```python
from build123d import *

# Parameters (mm, degrees)
EXTRUDE_1_DEPTH     = 17
EXTRUDE_2_DEPTH     = 2
SKETCH_4_R          = 3.35
EXTRUDE_3_DEPTH     = 5
SKETCH_5_R          = 1.7
EXTRUDE_4_DEPTH     = 6.8
CUT_EXTRUDE_1_DEPTH = 5


with BuildPart() as part:
    # Эскиз1 → Бобышка-Вытянуть1 (new body)
    with BuildSketch(Plane(origin=(0, 0, 0), x_dir=(0, 0, -1), z_dir=(1, 0, 0))):
        with BuildLine():
            Line((-3.35, -2.3), (-3.35, 2.3))
            ThreePointArc((-3.35, 2.3), (0, 5.65), (3.35, 2.3))
            Line((3.35, 2.3), (3.35, -2.3))
            ThreePointArc((3.35, -2.3), (0, -5.65), (-3.35, -2.3))
        make_face()
    extrude(amount=-EXTRUDE_1_DEPTH)

    # Эскиз3 → Бобышка-Вытянуть2 (add)
    with BuildSketch(Plane.ZY):
        with BuildLine():
            Line((2.15, 2.35), (2.15, -2.35))
            ThreePointArc((2.15, -2.35), (0, -4.5), (-2.15, -2.35))
            Line((-2.15, -2.35), (-2.15, 2.35))
            ThreePointArc((-2.15, 2.35), (0, 4.5), (2.15, 2.35))
        make_face()
    extrude(amount=-EXTRUDE_2_DEPTH)

    # Эскиз4 → Бобышка-Вытянуть3 (add)
    with BuildSketch(Plane(origin=(-17, 0, 0), x_dir=(0, 0, -1), z_dir=(1, 0, 0))):
        Circle(SKETCH_4_R)
    extrude(amount=-EXTRUDE_3_DEPTH)

    # По траектории1: sweep along a path in Эскиз6
    with BuildLine(Plane.XY) as sweep_1_path:
        Line((-22, 0), (-24.776161806, 0))
        ThreePointArc((-24.776161806, 0), (-30.870449905, -0.986593903), (-36.342181829, -3.845591055))
    # Эскиз5 → По траектории1 (sweep)
    with BuildSketch(Plane.ZY.offset(22)):
        Circle(SKETCH_5_R)
    sweep(path=sweep_1_path.line)

    # Эскиз7 → Бобышка-Вытянуть4 (add)
    with BuildSketch(Plane(origin=(2, 0, 0), x_dir=(0, 0, -1), z_dir=(1, 0, 0))):
        with BuildLine():
            Line((-1.2, -2.925), (-1.2, 2.925))
            ThreePointArc((-1.2, 2.925), (0, 4.125), (1.2, 2.925))
            Line((1.2, 2.925), (1.2, -2.925))
            ThreePointArc((1.2, -2.925), (0, -4.125), (-1.2, -2.925))
        make_face()
    extrude(amount=EXTRUDE_4_DEPTH)

    # Эскиз8 → Вырез-Вытянуть1 (cut)
    with BuildSketch(Plane(origin=(8.8, 0, -8.8), x_dir=(0, 0, 1), z_dir=(-1, 0, 0))):
        with BuildLine():
            Line((8.25, -3.15), (8.25, 3.15))
            ThreePointArc((8.25, 3.15), (8.8, 3.7), (9.35, 3.15))
            Line((9.35, 3.15), (9.35, -3.15))
            ThreePointArc((9.35, -3.15), (8.8, -3.7), (8.25, -3.15))
        make_face()
    extrude(amount=CUT_EXTRUDE_1_DEPTH, mode=Mode.SUBTRACT)


solid = part.part
```
Input: part model. Units: mm. Frame: model coordinates. A direction names the side the tool comes from. Round coordinates to 2 decimals unless told otherwise and drop trailing zeros. Loops run counter-clockwise (first coordinate to the right, second up) from the corner with the lowest first, then second, coordinate; pieces in that order, holes last. Notation, with made-up numbers: (66.25, 3.5) -> (71.25, 3.5) arc R18 ccw to (71.25, 32.5) -> close; hole circle Ø5 at (40, -31.5). An arc over 180 degrees is marked (long way). Use one line per item in the form item = value. Start each with the question number.
Item 1: Mould query, pull axis Y, two halves, no side actions, for faces 1 (the face through (-23.41, -1.66, -0.37)), 2 (the face through (-8.38, -5.65, -0.07)), 3 (the face through (8.8, 0, -1)), 4 (the face through (6.3, 3.7, 0)). Classes: pulls with the +Y half, pulls with the -Y half, needs draft (parallel to the pull), parting line crosses it, or undercut.
Item 2: Section query B-B on x = -4. Return the cut outline in (y, z), then the cut area to 3 significant figures.
Item 3: Section query A-A on z = 0. Return the cut outline in (x, y) (3 decimals).
Item 4: Contact query for flat-ended pins moving along their axis: pin 1 Ø4.5 at (x, y) = (6, -0.5) entering from -Z; pin 2 Ø2.5 at (x, y) = (6, -1) entering from +Z; pin 3 Ø0.9 at (y, z) = (-1.5, 0) entering from +X. Output: stop coordinate, or through.
Item 5: Material intervals for L1, parallel to Z at x = 4, y = -2.5; L2, parallel to Z at x = 2.5, y = -2.75; L3, parallel to X at y = 0.75, z = 2.75, sorted ascending. Write a range as from..to.
Item 6: Set-up query: faces 5 (the face through (1, 4.5, 0)), 6 (the face through (-22, 1, 2)), 7 (the face through (5, 0, -1.2)), 8 (the face through (6.3, -3.7, 0)), 9 (the face through (1, 0, 2.15)). Return all of +Z, -Z, +X, -X, +Y, -Y with unobstructed straight access to the full face (end or side cutting, diameter ignored); none if empty.
Ans:
q1.face_1 = parting line crosses it
q1.face_2 = pulls with the -Y half
q1.face_3 = needs draft
q1.face_4 = undercut
q2.outline = (-2.3, -3.35) -> (2.3, -3.35) arc R3.35 ccw to (2.3, 3.35) -> (-2.3, 3.35) arc R3.35 ccw to start
q2.area = 66.1 mm^2
q3.outline = (-37.36, -2.484) -> (-35.324, -5.207) arc R17.616 cw to (-24.776, -1.7) -> (-22, -1.7) -> (-22, -3.35) -> (-17, -3.35) -> (-17, -5.65) -> (0, -5.65) -> (0, -4.5) -> (2, -4.5) -> (2, -4.125) -> (8.8, -4.125) -> (8.8, -3.7) -> (3.8, -3.7) -> (3.8, 3.7) -> (8.8, 3.7) -> (8.8, 4.125) -> (2, 4.125) -> (2, 4.5) -> (0, 4.5) -> (0, 5.65) -> (-17, 5.65) -> (-17, 3.35) -> (-22, 3.35) -> (-22, 1.7) -> (-24.776, 1.7) arc R21.016 ccw to start
q4.pin_1 = -1.2
q4.pin_2 = 1.2
q4.pin_3 = 3.8
q5.L1 = -1.2..-0.55, 0.55..1.2
q5.L2 = -1.2..1.2
q5.L3 = -22..0
q6.face_5 = +X, +Y
q6.face_6 = none
q6.face_7 = -Z, +X, +Y, -Y
q6.face_8 = +X
q6.face_9 = +Z, +X, +Y, -Y
